```python
from build123d import *

# Parameters (mm, degrees)
ESBO_O1_R                = 1.625
ESBO_O1_R_2              = 3
ESBO_O1_W                = 41
ESBO_O1_H                = 21
RESSALTO_EXTRUS_O1_DEPTH = 3


with BuildPart() as part:
    # Esboço1 → Ressalto-extrusão1 (new body)
    with BuildSketch(Plane.XY):
        Polygon((215, -20), (160, -20), (160, -17), (130, -17), (130, -20), (80, -20), (80, -17), (50, -17), (50, -20), (0, -20), (0, 0), (179, 0), (179, 20), (250, 20), (250, -20), (250, -70.5), (215, -70.5), align=None)
        with Locations((189.8, 6.3)):
            Circle(ESBO_O1_R, mode=Mode.SUBTRACT)
        with Locations((239.2, 6.3)):
            Circle(ESBO_O1_R, mode=Mode.SUBTRACT)
        with Locations((239.2, -6.3)):
            Circle(ESBO_O1_R, mode=Mode.SUBTRACT)
        with Locations((189.8, -6.3)):
            Circle(ESBO_O1_R, mode=Mode.SUBTRACT)
        with Locations((232.5, -60.5)):
            Circle(ESBO_O1_R_2, mode=Mode.SUBTRACT)
        with Locations((232.5, -44.5)):
            Circle(ESBO_O1_R_2, mode=Mode.SUBTRACT)
        with Locations((214.5, 0)):
            Rectangle(ESBO_O1_W, ESBO_O1_H, mode=Mode.SUBTRACT)
        with BuildLine():
            Line((124, -6.5), (159, -6.5))
            ThreePointArc((159, -6.5), (160.5, -8), (159, -9.5))
            Line((159, -9.5), (124, -9.5))
            ThreePointArc((124, -9.5), (122.5, -8), (124, -6.5))
        make_face(mode=Mode.SUBTRACT)
    extrude(amount=RESSALTO_EXTRUS_O1_DEPTH)


solid = part.part
```
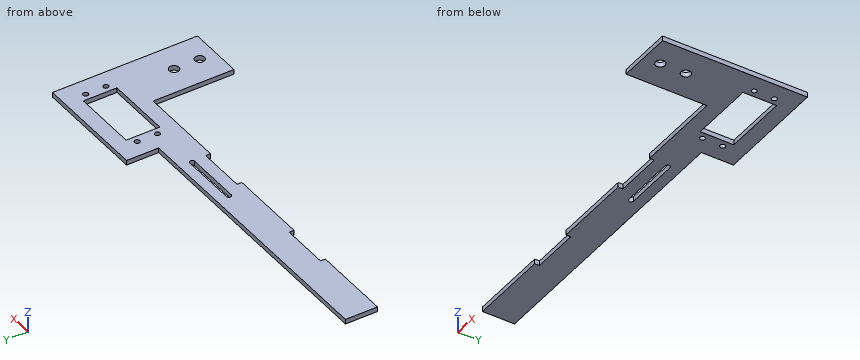
Geometry: final body of the model. Coordinates: model frame, mm. Coordinates: 2 decimals unless noted, no trailing zeros. Order: outer loops, then holes, each group sorted by start corner. A loop starts at its lowest first (then second) coordinate and runs counter-clockwise, first axis right, second up. Notation, with made-up numbers: M -4,60.25 L 29,60.25 A30 ccw 29,98.25 Z; hole C 6.5,-13 d8. An arc over 180 degrees is marked long. Answer as CSV lines item,"result".
Q1. Section A-A on x = 207.5. Return the cut outline in (y, z), and give its area (3 significant figures).
Answers:
outline,"M -20,0 L -10.5,0 L -10.5,3 L -20,3 Z; M 10.5,0 L 20,0 L 20,3 L 10.5,3 Z"
area,"57.0 mm^2"
Q2. First-contact query: P1, Ø1.5, axis at x = 107.5, z = 1, coming from the +Y side; P2, Ø1, axis at x = 91, z = 2.5, coming from the -Y side. Flat tips, straight axial feed; report the tip coordinate or a pass-through.
Answers:
P1,"stops at y = 0"
P2,"stops at y = -20"
Q3. Section C-C on z = 2.15. Count the separate pieces of the cut face and the enclosed holes in it, and give its area (3 significant figures).
Answers:
separate pieces,"1"
enclosed holes,"8"
area,"6,940 mm^2"
Q4. Section B-B on y = -60.5. Return the cut outline in (x, z).
Answers:
outline,"M 215,0 L 229.5,0 L 229.5,3 L 215,3 Z; M 235.5,0 L 250,0 L 250,3 L 235.5,3 Z"
Q5. Section D-D on y = -36.5. Return the cut outline in (x, z), and give its area (3 significant figures).
Answers:
outline,"M 215,0 L 250,0 L 250,3 L 215,3 Z"
area,"105 mm^2"
Q6. Line query: probe 1 along Y at (x, z) = (232.5, 1.3); probe 2 along Y at (x, z) = (239.2, 2.2) (3 decimals); probe 3 along X at (y, z) = (1.5, 0.45). Output: solid intervals per line, ascending. Write a range as [from, to].
Answers:
probe 1,"y = [-70.5, -63.5], [-57.5, -47.5], [-41.5, -10.5], [10.5, 20]"
probe 2,"y = [-70.5, -7.925], [-4.675, 4.675], [7.925, 20]"
probe 3,"x = [179, 194], [235, 250]"
